Part model, mm, in its own coordinate system. Face numbers are marked on the shaded views. A direction names the side the tool comes from. Coordinates: 2 decimals unless noted, no trailing zeros. Order: outer loops, then holes, each group sorted by start corner. A loop starts at its lowest first (then second) coordinate and runs counter-clockwise, first axis right, second up. Notation, with made-up numbers: M 12.25,76 L 64.25,76 A16 ccw 64.25,92 Z; hole C 8.25,78.25 d5. An arc over 180 degrees is marked long. Write item = value, one per line. Start each with the question number.
Autodesk Inventor part; units mm, degrees
ref_plane "YZ Plane" through (0, 0, 0) normal (1, 0, 0) x (0, 1, 0)
ref_plane "XZ Plane" through (0, 0, 0) normal (0, 1, 0) x (-1, 0, 0)
ref_plane "XY Plane" through (0, 0, 0) normal (0, 0, 1) x (1, 0, 0)
sketch "Sketch1" plane through (0, 0, 0) normal (0, 0, 1) x (1, 0, 0)
  circle A0 centre (0, 0) radius 3.75
  line L0 (-10, 20) -> (10, 20)
  line L1 (10, 20) -> (10, -20)
  line L2 (10, -20) -> (-10, -20)
  line L3 (-10, -20) -> (-10, 20)
  line L4 (-10, 20) -> (10, -20) construction
  line L5 (10, 20) -> (-10, -20) construction
  dimension "d0" = 7.5
  dimension "d1" = 40
  dimension "d2" = 20
extrude "Extrusion1" add sketch "Sketch1" along normal blind 4
sketch "Sketch2" plane through (-10, 20, 0) normal (0, 1, 0) x (1, 0, 0)
  line L0 (20, -4) -> (0, -4)
  line L1 (0, -4) -> (20, -4)
  line L2 (20, -4) -> (20, 20)
  line L3 (20, 20) -> (0, 20)
  line L4 (0, 20) -> (0, -4)
  point P0 (10, 0)
  dimension "d5" = 24
extrude "Extrusion2" add sketch "Sketch2" along normal blind 4
sketch "Sketch3" plane through (10, -20, 4) normal (1, 0, 0) x (0, 0, -1)
  line L0 (4, 0) -> (0, 0)
  line L1 (4, 40) -> (24, 40)
  line L2 (4, 0) -> (24, 40)
  line L3 (24, 40) -> (24, 44)
  line L4 (24, 40) -> (24, 44)
  line L5 (24, 44) -> (0, 44)
  line L6 (24, 44) -> (0, 44)
  line L7 (0, 0) -> (0, 44)
  line L8 (0, 44) -> (0, 0)
  line L9 (0, 0) -> (4, 0)
  point P0 (4, 20)
extrude "Extrusion3" add sketch "Sketch3" along normal blind 4
ref_plane "Work Plane1" through (0, -20, 4) normal (1, 0, 0) x (0, 0, -1)
mirror "Mirror1" about plane through (0, -20, 4) normal (1, 0, 0) of "Extrusion3"
sketch "Sketch4" plane through (14, 20, -20) normal (0, 0, -1) x (-1, 0, 0)
  line L0 (3.5, 0) -> (24.5, 0)
  line L1 (24.5, 0) -> (24.5, -40)
  line L2 (24.5, -40) -> (3.5, -40)
  line L3 (3.5, -40) -> (3.5, 0)
  line L4 (3.5, 0) -> (24.5, -40) construction
  line L5 (24.5, 0) -> (3.5, -40) construction
  point P0 (14, -20)
  dimension "d11" = 21
  dimension "d12" = 40
extrude "Extrusion4" cut sketch "Sketch4" against normal blind 20
properties part number "Gabarito Furo BOX 20"
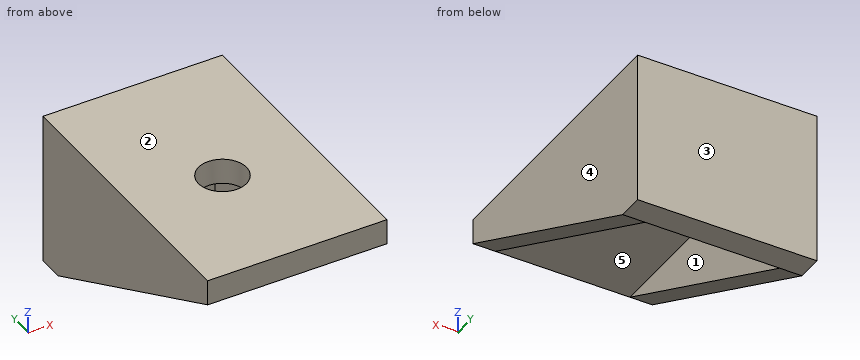
Item 1: Cut at C-C, the plane y = 18. Write the cut outline in (x, z), and give its area (3 significant figures).
Item 2: Cut at A-A, the plane x = 0. Write the cut outline in (y, z).
Item 3: Wall check: line 1 along X through (y, z) = (19, -12); line 2 along Y through (x, z) = (0, 1.8); line 3 along Y through (x, z) = (6.75, -0.5). Give the ranges that are in metal, low to high. Write a range as [from, to].
Item 4: Flat gauge pins, fed straight in: pin 1 (1.5 mm diameter, centred on x = 4.5, y = 18.5, fed in from -Z); pin 2 (10 mm diameter, centred on x = 2.5, z = -14.5, fed in from -Y). Where does each tip first touch, or does it go through?
Item 5: Cut at B-B, the plane y = 0. Write the cut outline in (x, z), and give its area (3 significant figures).
Item 6: Cut at D-D, the plane z = -8.25. Write the cut outline in (x, y), and give its area (4 significant figures).
Item 7: 3-axis set-ups, long thin cutter, end or side, ignore diameter. For the marked faces 1 and 2: which of +Z, -Z, +X, -X, +Y, -Y reach the whole face in a straight line?
Item 8: Pull direction X, two halves, no side cores. Call the marked faces 3, 4 and 5: pulls with the +X half, pulls with the -X half, needs draft (parallel to the pull), parting line crosses it, or undercut.
Filled sheet:
q1.outline = M -14,-19 L -10.5,-19 L -10.5,0 L 10.5,0 L 10.5,-19 L 14,-19 L 14,4 L -14,4 Z
q1.area = 245 mm2
q2.outline = M -20,0 L -3.75,0 L -3.75,4 L -20,4 Z; M 3.75,0 L 20,0 L 20,-20 L 24,-20 L 24,4 L 3.75,4 Z
q3.line_1 = [-14, -10.5], [10.5, 14]
q3.line_2 = [-20, -3.75], [3.75, 24]
q3.line_3 = [20, 24]
q4.pin_1 = 0
q4.pin_2 = 20
q5.outline = M -14,-10 L -10.5,-10 L -10.5,0 L -3.75,0 L -3.75,4 L -14,4 Z; M 3.75,0 L 10.5,0 L 10.5,-10 L 14,-10 L 14,4 L 3.75,4 Z
q5.area = 152 mm2
q6.outline = M -14,-3.5 L -10.5,-3.5 L -10.5,20 L 10.5,20 L 10.5,-3.5 L 14,-3.5 L 14,24 L -14,24 Z
q6.area = 276.5 mm2
q7.face_1 = -Z, -Y
q7.face_2 = +Z, +X, -X, +Y, -Y
q8.face_3 = needs draft
q8.face_4 = pulls with the +X half
q8.face_5 = undercut
